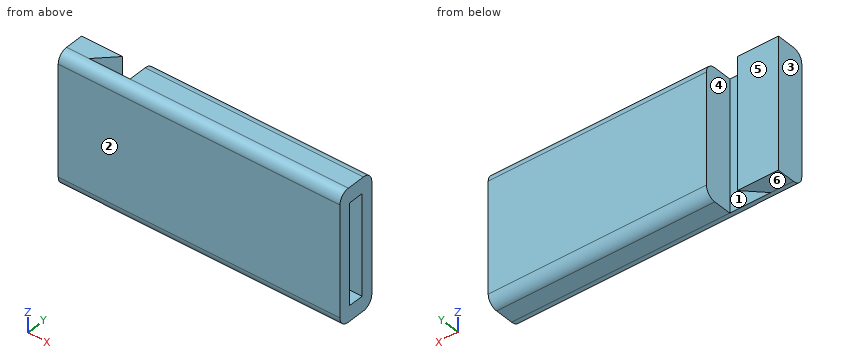
```python
from build123d import *

# Parameters (mm, degrees)
SKETCH1_W           = 55
SKETCH1_H           = 25.6
BOSS_EXTRUDE1_DEPTH = 7.6
CUT_EXTRUDE1_DEPTH  = 25.6
FILLET1_R           = 2
SKETCH3_W           = 19.6
SKETCH3_H           = 3
CUT_EXTRUDE2_DEPTH  = 10


with BuildPart() as part:
    # Sketch1 → Boss-Extrude1 (new body)
    with BuildSketch(Plane(origin=(0, 0, 0), x_dir=(1, 0, 0), z_dir=(0, 1, 0))):
        with Locations((27.5, 12.8)):
            Rectangle(SKETCH1_W, SKETCH1_H)
    extrude(amount=BOSS_EXTRUDE1_DEPTH)

    # Sketch2 → Cut-Extrude1 (cut)
    with BuildSketch(Plane(origin=(0, 0, -25.6), x_dir=(-1, 0, 0), z_dir=(0, 0, -1))):
        Polygon((-8, 5.6), (-4.4, 2), (-12.4, 2), (-12.4, 7.6), (0, 7.6), (0, 5.6), align=None)
    extrude(amount=-CUT_EXTRUDE1_DEPTH, mode=Mode.SUBTRACT)

    # Fillet1
    fillet1_edges = [part.edges().sort_by_distance(p)[0] for p in [
        (33.7, 7.6, -25.6),
        (33.7, 7.6, 0),
        (27.5, 0, -25.6),
        (27.5, 0, 0),
    ]]
    fillet(fillet1_edges, radius=FILLET1_R - 0.0001)  # a hair under: the kernel refuses the full size

    # Sketch3 → Cut-Extrude2 (cut)
    with BuildSketch(Plane(origin=(55, 0, 0), x_dir=(0, 0, -1), z_dir=(1, 0, 0))):
        with Locations((12.8, 3.8)):
            Rectangle(SKETCH3_W, SKETCH3_H)
    extrude(amount=-CUT_EXTRUDE2_DEPTH, mode=Mode.SUBTRACT)


solid = part.part
```
The model under review builds one solid part; all positions refer to its coordinate system, in mm. Face numbers are marked on the shaded views. A direction names the side the tool comes from. Round coordinates to 2 decimals unless told otherwise and drop trailing zeros. Write each loop counter-clockwise with the first axis right and the second up, starting at its lowest first coordinate (ties: lowest second). Pieces come first, ordered by that corner, then holes. Notation, with made-up numbers: (-30.75, 49) - (19.25, 49) arc R15 cw to (19.25, 60) - close; hole circle Ø2 at (58.25, 78.5). An arc over 180 degrees is marked (long way). Use one line per item in the form item = value.
Q1. Insertion check: pin 1 Ø2.5 at (x, z) = (8.5, -8) entering from +Y. The pin has a flat end and moves straight along its axis. Give the tip position at first contact, or say it passes through.
Answer key:
pin_1 = 5.6
Q2. For line 1 (Y direction, x = 46, z = -5); line 2 (Z direction, x = 47.5, y = 4.25); line 3 (Y direction, x = 7, z = -21.75), list the stretches that pass through material, from the lowest coordinate up. Write a range as [from, to].
Answer key:
line_1 = [0, 2.3], [5.3, 7.6]
line_2 = [-25.6, -22.6], [-3, 0]
line_3 = [0, 2], [4.6, 5.6]
Q3. Consider section D-D (y = 0.5). State the section outline as (x, z) points.
Answer key:
outline = (0, -24.92) - (55, -24.92) - (55, -0.68) - (0, -0.68) - close
Q4. Tool access review of the marked faces 4, 5 and 6: name each direction out of +Z, -Z, +X, -X, +Y, -Y from which nothing blocks a thin tool from reaching the whole face with its end or side.
Answer key:
face_4 = +Z, -Z, +Y
face_5 = +Z, -Z, -X, +Y
face_6 = -Z, +X, -X, +Y, -Y
Q5. Consider section B-B (z = -5.25). State the section outline as (x, y) points.
Answer key:
outline = (0, 0) - (55, 0) - (55, 2.3) - (45, 2.3) - (45, 5.3) - (55, 5.3) - (55, 7.6) - (12.4, 7.6) - (12.4, 2) - (4.4, 2) - (8, 5.6) - (0, 5.6) - close
Q6. Draft analysis for pull direction X (two halves, no side actions). For the marked faces 1, 2 and 3, state which applies: +X half, -X half, draft (parallel to the pull), parting line (faces both ways), or undercut.
Answer key:
face_1 = undercut
face_2 = draft
face_3 = -X half
Q7. Consider section A-A (x = 47.5). State the section outline as (y, z) points.
Answer key:
outline = (0, -23.6) arc R2 ccw to (2, -25.6) - (5.6, -25.6) arc R2 ccw to (7.6, -23.6) - (7.6, -2) arc R2 ccw to (5.6, 0) - (2, 0) arc R2 ccw to (0, -2) - close; hole (2.3, -22.6) - (5.3, -22.6) - (5.3, -3) - (2.3, -3) - close
Q8. Consider section C-C (x = 19). State the section outline as (y, z) points, and give its area (3 significant figures).
Answer key:
outline = (0, -23.6) arc R2 ccw to (2, -25.6) - (5.6, -25.6) arc R2 ccw to (7.6, -23.6) - (7.6, -2) arc R2 ccw to (5.6, 0) - (2, 0) arc R2 ccw to (0, -2) - close
area = 191 mm2
